Could you check a few things on this model? Use its own coordinates, in mm. A direction names the side the tool comes from. Coordinates: 2 decimals unless noted, no trailing zeros. Write each loop counter-clockwise with the first axis right and the second up, starting at its lowest first coordinate (ties: lowest second). Pieces come first, ordered by that corner, then holes. Notation, with made-up numbers: (88.5, 15.25) - (133.5, 15.25) arc R20 cw to (133.5, 52.25) - close; hole circle Ø5 at (52, 27.5). An arc over 180 degrees is marked (long way). Answer as a JSON object with one key per item and string values. Group by question number.
1) If we section it at A-A (y = -3.5): Write out the boundary of the cut face in (x, z).
2) If we section it at B-B (z = -24.25): State how many separate pieces and enclosed holes the cut face has, plus the area to 3 significant figures.
3) If we section it at C-C (y = 14): Write out the boundary of the cut face in (x, z).
4) On a 3-axis mill with a long thin cutter (end or side, diameter ignored), from which of +Z, -Z, +X, -X, +Y, -Y can I reach the whole of each face in a straight line? I mean faces 1 (the cylindrical face through (28.088, -13.137, -24.535)), 2 (the cylindrical face through (21.555, -6.28, -24.535)). Say none if no direction works.
5) Please list where these lines run through material, in increasing order: line 1 along X through (y, z) = (-0.5, -24.65); line 2 along Y through (x, z) = (0, -23.35); line 3 along Y through (x, z) = (44, -25.7).
6) Will these pins go through, and if not, where does the flat tip stop? pin 1 Ø1.8 at (x, y) = (30.19, -33.37) entering from -Z; pin 2 Ø2 at (y, z) = (6, -26) entering from +X; pin 3 Ø1.5 at (x, z) = (1.5, -23) entering from +Y; pin 4 Ø3 at (x, z) = (10.5, -25) entering from +Y.
7) We'd pull the mould along X, two halves only. Please class faces 3 (the flat face through (33.95, -35.71, -24.54)), 4 (the flat face through (24.612, 34.566, -24.535)), 5 (the flat face through (6.56, -13.02, -24.54)): released by +X, released by -X, zero draft, split by the parting line, or undercut.
```python
from build123d import *

# Parameters (mm, degrees)
SKETCH2_R           = 1.5
BOSS_EXTRUDE1_DEPTH = 5
FILLET1_R           = 2


with BuildPart() as part:
    # Sketch2 → Boss-Extrude1 (new body)
    with BuildSketch(Plane(origin=(6.301928067, 33.341579781, -27), x_dir=(-0.670801619, 0.74163683, 0), z_dir=(0, 0, -1))):
        with BuildLine():
            Line((-60.01425581, -23.839998272), (-68.549452032, -21.468875235))
            Line((-68.549452032, -21.468875235), (-70.98574419, -30.238657023))
            Line((-70.98574419, -30.238657023), (-62.450547968, -32.60978006))
            Line((-62.450547968, -32.60978006), (-39.815769516, -40.315756269))
            Line((-39.815769516, -40.315756269), (-25.661547731, -39.280246834))
            Line((-25.661547731, -39.280246834), (-18.621605657, -30.094798604))
            Line((-18.621605657, -30.094798604), (-9.456704001, -17.167000829))
            Line((-9.456704001, -17.167000829), (-5.335690467, 4.468320227))
            Line((-5.335690467, 4.468320227), (-17.584258472, 24.615497506))
            Line((-17.584258472, 24.615497506), (-22.792310688, 26.388571034))
            Line((-22.792310688, 26.388571034), (-37.355145596, 31.346466229))
            Line((-37.355145596, 31.346466229), (-53.38998859, 22.351505712))
            Line((-53.38998859, 22.351505712), (-53.38998859, 11.040844476))
            Line((-53.38998859, 11.040844476), (-48.457282179, -4.144818068))
            ThreePointArc((-48.457282179, -4.144818068), (-49.150509534, -15.1642744), (-57.197834388, -22.724006186))
            Line((-57.197834388, -22.724006186), (-60.01425581, -23.839998272))
        make_face()
        with Locations((-65.5, -27.039327647)):
            Circle(SKETCH2_R, mode=Mode.SUBTRACT)
        with Locations((-20.5, -27.039327647)):
            Circle(SKETCH2_R, mode=Mode.SUBTRACT)
        with Locations((-15.8, 11.676431418)):
            Circle(SKETCH2_R, mode=Mode.SUBTRACT)
        with BuildLine():
            Line((-47.130315082, -28.318253081), (-38.647453771, -31.206230429))
            Line((-38.647453771, -31.206230429), (-30.347341702, -30.599002106))
            Line((-30.347341702, -30.599002106), (-25.866841879, -24.753016622))
            Line((-25.866841879, -24.753016622), (-17.931352522, -13.559399331))
            Line((-17.931352522, -13.559399331), (-14.824551002, 2.751308649))
            Line((-14.824551002, 2.751308649), (-23.577444554, 17.1485915))
            Line((-23.577444554, 17.1485915), (-25.692860174, 17.86878156))
            Line((-25.692860174, 17.86878156), (-36.454250771, 21.532480769))
            Line((-36.454250771, 21.532480769), (-44.38998859, 17.080822067))
            Line((-44.38998859, 17.080822067), (-44.38998859, 12.465915799))
            Line((-44.38998859, 12.465915799), (-39.897539246, -1.364386282))
            ThreePointArc((-39.897539246, -1.364386282), (-39.671812155, -15.458597607), (-47.39803378, -27.248561347))
            Line((-47.39803378, -27.248561347), (-47.130315082, -28.318253081))
        make_face(mode=Mode.SUBTRACT)
    extrude(amount=-BOSS_EXTRUDE1_DEPTH)

    # Fillet1
    fillet1_edges = [part.edges().sort_by_distance(p)[0] for p in [
        (31.493178432, -39.588202626, -24.5),
        (36.362902877, -31.898574812, -24.5),
    ]]
    fillet(fillet1_edges, radius=FILLET1_R)


solid = part.part
```
Here are the results:
{
 "1": {"outline": "(-4.05, -27) - (5.1, -27) - (5.1, -22) - (-4.05, -22) - close; (23.6, -27) - (39.92, -27) - (39.92, -22) - (23.6, -22) - close"},
 "2": {"separate pieces": "1", "enclosed holes": "4", "area": "1,680 mm²"},
 "3": {"outline": "(-0.27, -27) - (10.58, -27) - (10.58, -22) - (-0.27, -22) - close; (48.26, -27) - (57.49, -27) - (57.49, -22) - (48.26, -22) - close"},
 "4": {"face 1": "+Z, -Z, +X", "face 2": "+Z, -Z"},
 "5": {"line 1": "x = -3.49 to -1.41, 1.41 to 5.73, 26.66 to 46.62", "line 2": "y = -19.24 to -1.5, 1.5 to 14.93", "line 3": "y = -1.67 to 8.19, 22.26 to 32.56"},
 "6": {"pin 1": "passes through", "pin 2": "stops at x = 56.77", "pin 3": "stops at y = 17.9", "pin 4": "stops at y = 30.8"},
 "7": {"face 3": "released by +X", "face 4": "released by -X", "face 5": "undercut"}
}
